```python
from build123d import *

# Parameters (mm, degrees)
F0_W     = 45
F0_H     = 8
F0_W_2   = 16
F0_R     = 4
F0_H_2   = 2
F1_DEPTH = 15
F2_R     = 3
F3_DEPTH = 55.5


# Not quite as in the source:
# - a feature names something its author has since deleted; it is built from what else it names


with BuildPart() as f1:
    # F0 (on Front) → F1 (new body)
    with BuildSketch(Plane.XZ):
        with Locations((22.5, 4)):
            Rectangle(F0_W, F0_H)
        with Locations((53, 4)):
            Rectangle(F0_W_2, F0_H)
        Polygon((45, 40.5), (45, 8), (61, 8), (61, 46), (45, 46), align=None)
        with Locations((53, 38)):
            Circle(F0_R, mode=Mode.SUBTRACT)
        Polygon((39, 40.5), (45, 40.5), (45, 46), (45, 48), (39, 48), align=None)
        with Locations((53, 47)):
            Rectangle(F0_W_2, F0_H_2)
    extrude(amount=F1_DEPTH)

    # F2 (on face) → F3 (cut, symmetric)
    with BuildSketch(Plane.XY.offset(8)):
        with Locations((10, -7.5)):
            Circle(F2_R)
    extrude(amount=F3_DEPTH, both=True, mode=Mode.SUBTRACT)


solid = f1.part
```
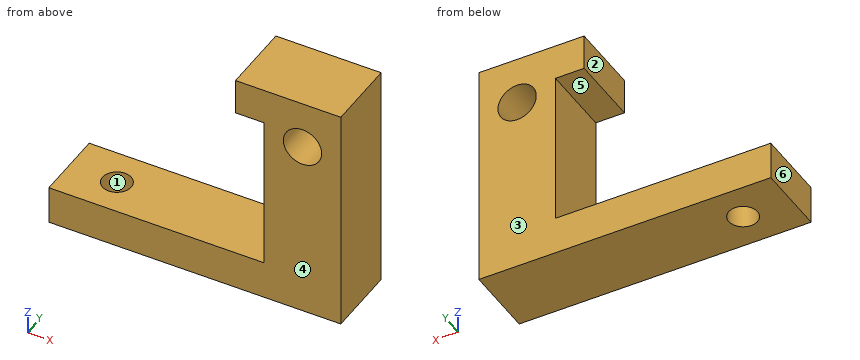
For this review, take the finished solid that the model builds, in its own axes (mm). Face numbers are marked on the shaded views. A direction names the side the tool comes from. Round coordinates to 2 decimals unless told otherwise and drop trailing zeros. Write each loop counter-clockwise with the first axis right and the second up, starting at its lowest first coordinate (ties: lowest second). Pieces come first, ordered by that corner, then holes. Notation, with made-up numbers: (52.25, -33) -> (82.25, -33) arc R17 ccw to (82.25, -2) -> close; hole circle Ø8 at (57.25, -10.5). An arc over 180 degrees is marked (long way). One line per question, with ' | ' between items. Start each with the question number.
1) Add section B-B (y = -7.5). Write out the cut boundary in (x, z), and give its area (3 significant figures).
2) Add section C-C (z = 38). Write out the cut boundary in (x, y).
3) Machinability: for the marked faces 5 and 6, which of the approach directions +Z, -Z, +X, -X, +Y, -Y give a long, thin tool a straight path to every point of the face, cutting with its end or side? Answer none if there is none.
4) For pin 1 Ø4.5 at (x, y) = (23.5, -5) entering from +Z; pin 2 Ø4.5 at (y, z) = (-6, 19) entering from -X; pin 3 Ø4 at (y, z) = (-11, 46) entering from -X, all flat-tipped, find the tip position at first contact; note any pin that passes through.
5) Add section D-D (y = -2.5). Write out the cut boundary in (x, z).
6) Add section A-A (x = 10). Write out the cut boundary in (y, z), and give its area (3 significant figures).
7) Wall thickness on line 1 along Z through (x, y) = (42.5, -13); line 2 along X through (y, z) = (-7.25, 25.5); line 3 along Z through (x, y) = (53, -3): over which ranges is each line inside the solid? List them lowest first.
8) Mouldability with a two-part tool opening along Y and no side actions: class the marked faces 1, 2, 3 and 4 as +Y half, -Y half, draft (parallel to the pull), parting line (faces both ways), or undercut.
Reported:
1) outline: (0, 0) -> (7, 0) -> (7, 8) -> (0, 8) -> close; (13, 0) -> (61, 0) -> (61, 48) -> (39, 48) -> (39, 40.5) -> (45, 40.5) -> (45, 8) -> (13, 8) -> close; hole circle Ø8 at (53, 38) | area: 1,070 mm²
2) outline: (45, -15) -> (49, -15) -> (49, 0) -> (45, 0) -> close; (57, -15) -> (61, -15) -> (61, 0) -> (57, 0) -> close
3) face 5: -X, +Y, -Y | face 6: +Z, -Z, -X, +Y, -Y
4) pin 1: stops at z = 8 | pin 2: stops at x = 45 | pin 3: stops at x = 39
5) outline: (0, 0) -> (61, 0) -> (61, 48) -> (39, 48) -> (39, 40.5) -> (45, 40.5) -> (45, 8) -> (0, 8) -> close; hole circle Ø8 at (53, 38)
6) outline: (-15, 0) -> (-10.5, 0) -> (-10.5, 8) -> (-15, 8) -> close; (-4.5, 0) -> (0, 0) -> (0, 8) -> (-4.5, 8) -> close | area: 72.0 mm²
7) line 1: z = 0 to 8, 40.5 to 48 | line 2: x = 45 to 61 | line 3: z = 0 to 34, 42 to 48
8) face 1: undercut | face 2: draft | face 3: +Y half | face 4: -Y half
